Can you work these out from the model? Positions are in its coordinate system, mm. Face numbers are marked on the shaded views. A direction names the side the tool comes from. Coordinates: 2 decimals unless noted, no trailing zeros. Order: outer loops, then holes, each group sorted by start corner. A loop starts at its lowest first (then second) coordinate and runs counter-clockwise, first axis right, second up. Notation, with made-up numbers: (63.25, 37.5) -> (84.25, 37.5) arc R15 ccw to (84.25, 65.5) -> close; hole circle Ø4 at (85, -13). An arc over 180 degrees is marked (long way). Write item = value, one per line.
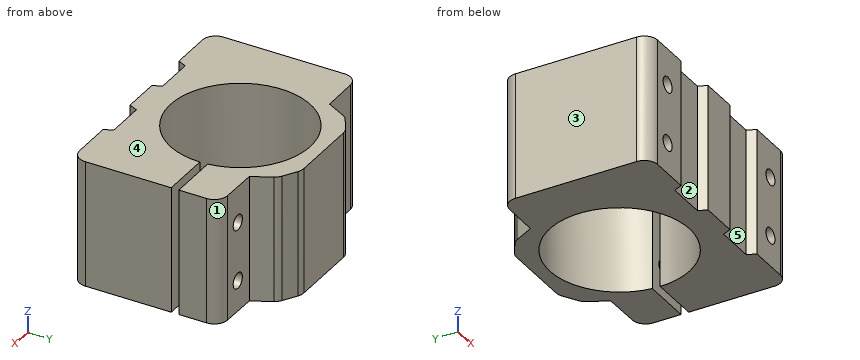
```python
from build123d import *

# Parameters (mm, degrees)
F2_DEPTH = 47
F0_R     = 2.88967587
F3_DEPTH = 69
F4_R     = 5
F5_SIZE  = 5
F6_R     = 5


with BuildPart() as f2:
    # F1 (on Top) → F2 (new body)
    with BuildSketch(Plane.XY):
        with BuildLine():
            Line((-7, 0), (0, 0))
            Line((0, 0), (7, 0))
            Line((7, 0), (8.4177446879, 3.2))
            Line((8.4177446879, 3.2), (22.9177446879, 3.2))
            Line((22.9177446879, 3.2), (24.3354893758, 0))
            Line((24.3354893758, 0), (44.3354893758, 0))
            Line((44.3354893758, 0), (44.3354893758, 37))
            Line((44.3354893758, 37), (26, 37))
            ThreePointArc((26, 37), (-25.9613897172, 35.5835805883), (25.8456735423, 39.8286320269))
            Line((25.8456735423, 39.8286320269), (44.3354893758, 39.8286320269))
            Line((44.3354893758, 39.8286320269), (44.3354893758, 55.0705678761))
            Line((44.3354893758, 55.0705678761), (25.764113456, 55.2520155907))
            Line((25.764113456, 55.2520155907), (19.0504045933, 68))
            Line((19.0504045933, 68), (-19.0504045933, 68))
            Line((-19.0504045933, 68), (-25.764113456, 55.2520155907))
            Line((-25.764113456, 55.2520155907), (-44.3354893758, 55.0705678761))
            Line((-44.3354893758, 55.0705678761), (-44.3354893758, 0))
            Line((-44.3354893758, 0), (-24.3354893758, 0))
            Line((-24.3354893758, 0), (-22.9177446879, 3.2))
            Line((-22.9177446879, 3.2), (-8.4177446879, 3.2))
            Line((-8.4177446879, 3.2), (-7, 0))
        make_face()
    extrude(amount=F2_DEPTH)

    # F0 (on Front) → F3 (cut)
    with BuildSketch(Plane.XZ):
        with Locations((-33, 33.5)):
            Circle(F0_R)
        with Locations((-33, 11.5)):
            Circle(F0_R)
        with Locations((33, 33.5)):
            Circle(F0_R)
        with Locations((33, 11.5)):
            Circle(F0_R)
    extrude(amount=-F3_DEPTH, mode=Mode.SUBTRACT)

    # F4
    f4_edges = [f2.edges().sort_by_distance(p)[0] for p in [
        (-44.335489, 55.070568, 23.5),
        (44.335489, 55.070568, 23.5),
    ]]
    fillet(f4_edges, radius=F4_R)

    # F5
    f5_edges = [f2.edges().sort_by_distance(p)[0] for p in [
        (19.050405, 68, 23.5),
        (-19.050405, 68, 23.5),
    ]]
    chamfer(f5_edges, length=F5_SIZE)

    # F6
    f6_edges = [f2.edges().sort_by_distance(p)[0] for p in [
        (21.38029, 63.576016, 23.5),
        (14.050405, 68, 23.5),
        (-14.050405, 68, 23.5),
        (-21.38029, 63.576016, 23.5),
        (44.335489, 0, 23.5),
        (-44.335489, 0, 23.5),
    ]]
    fillet(f6_edges, radius=F6_R)


solid = f2.part
```
Item 1: I want a section at B-B, the plane y = 22. Please give me the cut outline in (x, z).
A:
outline = (-44.34, 0) -> (-21.24, 0) -> (-21.24, 47) -> (-44.34, 47) -> close; (21.24, 0) -> (44.34, 0) -> (44.34, 47) -> (21.24, 47) -> close; hole circle Ø5.78 at (-33, 11.5); hole circle Ø5.78 at (-33, 33.5); hole circle Ø5.78 at (33, 11.5); hole circle Ø5.78 at (33, 33.5)
Item 2: I want a section at A-A, the plane x = 0. Please give me the cut outline in (y, z).
A:
outline = (0, 0) -> (11, 0) -> (11, 47) -> (0, 47) -> close; (63, 0) -> (68, 0) -> (68, 47) -> (63, 47) -> close
Item 3: I'm going to push flat-ended pins straight in: P1, Ø4.5, axis at x = 33, z = 33.5, coming from the +Y side; P2, Ø10, axis at x = 18, z = 37, coming from the +Y side; P3, Ø5.5, axis at x = 30.5, z = 32.5, coming from the +Y side; P4, Ø11.5, axis at x = -13.5, z = 24.5, coming from the -Y side. Where does each tip first touch, or does it pass through?
A:
P1 = through
P2 = 67.99
P3 = 55.23
P4 = 1.69
Item 4: If we mould it in two halves opening along X, with no side actions, what happens to the marked faces 1, 2 and 3? For each: pulls with the +X half, pulls with the -X half, needs draft (parallel to the pull), parting line crosses it, or undercut.
A:
face_1 = pulls with the +X half
face_2 = undercut
face_3 = pulls with the -X half
Item 5: I want a section at D-D, the plane x = -32.5. Please give me the cut outline in (y, z).
A:
outline = (0, 0) -> (55.19, 0) -> (55.19, 8.65) -> (0, 8.65) -> close; (0, 14.35) -> (55.19, 14.35) -> (55.19, 30.65) -> (0, 30.65) -> close; (0, 36.35) -> (55.19, 36.35) -> (55.19, 47) -> (0, 47) -> close
Item 6: For the marked faces 4 and 5, which set-ups out of +Z, -Z, +X, -X, +Y, -Y let a thin tool reach every point of the face, with its end or its side?
A:
face_4 = +Z, +X, -X, +Y, -Y
face_5 = +Z, -Z, -Y
Item 7: If I drill on probe 1 along Z at (x, y) = (-33, 43.5); probe 2 along Y at (x, z) = (0, 33); probe 3 along X at (y, z) = (50.25, 11.5), over which ranges is the centre line in solid material (lowest first)?
A:
probe_1 = 0 to 8.61, 14.39 to 30.61, 36.39 to 47
probe_2 = 0 to 11, 63 to 68
probe_3 = -44.33 to -35.89, -30.11 to -22.37, 22.37 to 30.11, 35.89 to 44.33
